from build123d import *

# Parameters (mm, degrees)
F0_R     = 11.1125
F0_R_2   = 6.0325
F0_R_3   = 4.318
F0_R_4   = 2.1082
F1_DEPTH = 5.08
F2_DEPTH = 10.414
F3_START = 4.445
F3_DEPTH = 8.255


with BuildPart() as f1:
    # F0 (on Right) → F1 (new body)
    with BuildSketch(Plane.YZ):
        Circle(F0_R)
        Circle(F0_R_2, mode=Mode.SUBTRACT)
        Circle(F0_R_2)
        Circle(F0_R_3, mode=Mode.SUBTRACT)
        Circle(F0_R_3)
        Circle(F0_R_4, mode=Mode.SUBTRACT)
    extrude(amount=F1_DEPTH)

    # F0 (on Right) → F2 (join)
    with BuildSketch(Plane.YZ):
        Circle(F0_R_2)
        Circle(F0_R_3, mode=Mode.SUBTRACT)
        Circle(F0_R_3)
        Circle(F0_R_4, mode=Mode.SUBTRACT)
    extrude(amount=F2_DEPTH)

    # F0 (on Right) → F3 (cut)
    with BuildSketch(Plane.YZ.offset(F3_START)):
        Circle(F0_R_3)
        Circle(F0_R_4, mode=Mode.SUBTRACT)
    extrude(amount=F3_DEPTH, mode=Mode.SUBTRACT)


solid = f1.part
Design review of the part built by this model. Coordinates are the model's own, in mm. A direction names the side the tool comes from. Round coordinates to 2 decimals unless told otherwise and drop trailing zeros. Loops run counter-clockwise (first coordinate to the right, second up) from the corner with the lowest first, then second, coordinate; pieces in that order, holes last. Notation, with made-up numbers: (88, 3.5) - (126, 3.5) arc R22 cw to (126, 37.5) - close; hole circle Ø7 at (82, 55). An arc over 180 degrees is marked (long way). One line per question, with ' | ' between items.
1. Clearance check with flat-ended pins moving along their axes: P1, Ø10, axis at y = -0.5, z = 1, coming from the -X side; P2, Ø1, axis at x = 3.5, y = 5.5, coming from the +Z side; P3, Ø1, axis at x = 4, y = -4.5, coming from the +Z side; P4, Ø4.5, axis at y = -0.5, z = -1, coming from the +X side (3 decimals). State where each tip first meets the part, or that it passes through.
Results are:
P1: stops at x = 0 | P2: stops at z = 9.92 | P3: stops at z = 10.37 | P4: stops at x = 4.445
2. For faces 1 (the face through (5.08, 5, -5)), 2 (the face through (0, -0.2, -2.3)), list the 3-axis set-ups (+Z, -Z, +X, -X, +Y, -Y) from which the entire face can be reached by the end or side of a thin tool; tool diameter is ignored.
Results are:
face 1: +X | face 2: +Z, -Z, -X, +Y, -Y
3. We need section D-D, the plane y = -3. State the section outline as (x, z) points (3 decimals).
Results are:
outline: (0, -10.7) - (5.08, -10.7) - (5.08, -5.234) - (10.414, -5.234) - (10.414, -3.106) - (4.445, -3.106) - (4.445, 3.106) - (10.414, 3.106) - (10.414, 5.234) - (5.08, 5.234) - (5.08, 10.7) - (0, 10.7) - close
4. Draft analysis for pull direction Z (two halves, no side actions). For faces 3 (the face through (7.71, 5.754, 1.812)), 4 (the face through (2.19, -0.27, 2.09)), 5 (the face through (7.39, -0.56, 4.28)), 6 (the face through (10.414, 3, -4)), state which applies: released by +Z, released by -Z, zero draft, split by the parting line, or undercut.
Results are:
face 3: split by the parting line | face 4: undercut | face 5: undercut | face 6: zero draft
5. We need section A-A, the plane z = 0. State the section outline as (x, y) points (1 decimal), and give its area (3 significant figures).
Results are:
outline: (0, -11.1) - (5.1, -11.1) - (5.1, -6) - (10.4, -6) - (10.4, -4.3) - (4.4, -4.3) - (4.4, -2.1) - (0, -2.1) - close; (0, 2.1) - (4.4, 2.1) - (4.4, 4.3) - (10.4, 4.3) - (10.4, 6) - (5.1, 6) - (5.1, 11.1) - (0, 11.1) - close | area: 107 mm²
6. We need section C-C, the plane x = 8.5. State the section outline as (y, z) points (1 decimal).
Results are:
outline: circle Ø12.1 at (0, 0); hole circle Ø8.6 at (0, 0)
7. For L1, parallel to Z at x = 2.3, y = 0; L2, parallel to Y at x = 5.5, z = 0, list the stretches that pass through material, from the lowest coordinate up. Write a range as [from, to].
Results are:
L1: z = [-11.11, -2.11], [2.11, 11.11] | L2: y = [-6.03, -4.32], [4.32, 6.03]
